The listing builds one solid part. Answer for the finished solid, in the listing's coordinates (mm). A direction names the side the tool comes from. Coordinates: 2 decimals unless noted, no trailing zeros. Order: outer loops, then holes, each group sorted by start corner. A loop starts at its lowest first (then second) coordinate and runs counter-clockwise, first axis right, second up. Notation, with made-up numbers: (68, 47.25) -> (91, 47.25) arc R30 cw to (91, 74.25) -> close; hole circle Ø2 at (7.5, -21). An arc over 180 degrees is marked (long way). Write item = value, one per line. Start each with the question number.
```python
from build123d import *

# Parameters (mm, degrees)
ESQUISSE1_W             = 69
ESQUISSE1_H             = 34
BOSS_EXTRU_1_DEPTH      = 140
COQUE1_T                = 3
CONG_3_R                = 4
ESQUISSE2_W             = 19
ESQUISSE2_H             = 10
ESQUISSE2_R             = 1.75
BOSS_EXTRU_2_DEPTH      = 4
CONG_5_R                = 3.5
ESQUISSE1_2_W           = 69
ESQUISSE1_2_H           = 34
ENL_V_MAT_EXTRU_1_DEPTH = 140
CONG_4_R                = 1
CONG_7_R                = 3
ENL_V_MAT_EXTRU_2_REACH = 155.64
ESQUISSE3_W             = 61
ESQUISSE3_H             = 26
CONG_8_R                = 1


with BuildPart() as part:
    # Esquisse1 → Boss.-Extru.1 (new body)
    with BuildSketch(Plane.XY):
        Rectangle(ESQUISSE1_W, ESQUISSE1_H)
    extrude(amount=BOSS_EXTRU_1_DEPTH)

    # Coque1
    coque1_openings = [part.faces().sort_by_distance(p)[0] for p in [
        (0, 0, 140),
    ]]
    offset(amount=COQUE1_T, openings=coque1_openings, kind=Kind.INTERSECTION)

    # Congé3
    # the kernel refuses this fillet: 4 mm, written as the material it takes off along each edge
    with BuildSketch(Plane(origin=(33.5, 16, 1), x_dir=(0, 1, 0), z_dir=(0, 0, -1))) as cong_3_piece_1_section:
        Polygon((0, 0), (CONG_3_R, 0), (CONG_3_R, CONG_3_R), (0, CONG_3_R), align=None)
    cong_3_piece_1 = extrude(amount=CONG_3_R, mode=Mode.PRIVATE)
    cong_3_piece_1 = cong_3_piece_1 - Plane(origin=(33.5, 16, 1), x_dir=(-0.7071067811865475, -0.7071067811865475, 0), z_dir=(0, 0, -1)) * Sphere(CONG_3_R, mode=Mode.PRIVATE)
    add(cong_3_piece_1, mode=Mode.SUBTRACT)
    with BuildSketch(Plane(origin=(-33.5, 16, 1), x_dir=(0, 0, -1), z_dir=(-1, 0, 0))) as cong_3_piece_2_section:
        Polygon((0, 0), (CONG_3_R, 0), (CONG_3_R, -CONG_3_R), (0, -CONG_3_R), align=None)
    cong_3_piece_2 = extrude(amount=CONG_3_R, mode=Mode.PRIVATE)
    cong_3_piece_2 = cong_3_piece_2 - Plane(origin=(-33.5, 16, 1), x_dir=(0, -0.7071067811865475, 0.7071067811865475), z_dir=(-1, 0, 0)) * Sphere(CONG_3_R, mode=Mode.PRIVATE)
    add(cong_3_piece_2, mode=Mode.SUBTRACT)
    with BuildSketch(Plane(origin=(33.5, -16, 1), x_dir=(0, 0, -1), z_dir=(0, -1, 0))) as cong_3_piece_3_section:
        Polygon((0, 0), (CONG_3_R, 0), (CONG_3_R, CONG_3_R), (0, CONG_3_R), align=None)
    cong_3_piece_3 = extrude(amount=CONG_3_R, mode=Mode.PRIVATE)
    cong_3_piece_3 = cong_3_piece_3 - Plane(origin=(33.5, -16, 1), x_dir=(-0.7071067811865475, 0, 0.7071067811865475), z_dir=(0, -1, 0)) * Sphere(CONG_3_R, mode=Mode.PRIVATE)
    add(cong_3_piece_3, mode=Mode.SUBTRACT)
    with BuildSketch(Plane(origin=(-33.5, -16, 1), x_dir=(-1, 0, 0), z_dir=(0, -1, 0))) as cong_3_piece_4_section:
        Polygon((0, 0), (CONG_3_R, 0), (CONG_3_R, CONG_3_R), (0, CONG_3_R), align=None)
    cong_3_piece_4 = extrude(amount=CONG_3_R, mode=Mode.PRIVATE)
    cong_3_piece_4 = cong_3_piece_4 - Plane(origin=(-33.5, -16, 1), x_dir=(0.7071067811865475, 0, 0.7071067811865475), z_dir=(0, -1, 0)) * Sphere(CONG_3_R, mode=Mode.PRIVATE)
    add(cong_3_piece_4, mode=Mode.SUBTRACT)
    with BuildSketch(Plane(origin=(33.5, 20, -3), x_dir=(0, 0, 1), z_dir=(-1, 0, 0)), Plane(origin=(-33.5, -20, -3), x_dir=(0, 0, 1), z_dir=(1, 0, 0))) as cong_3_piece_5:
        with BuildLine():
            CenterArc((CONG_3_R, -CONG_3_R), CONG_3_R, 90, 90)
            Line((0, -CONG_3_R), (0, 0))
            Line((0, 0), (CONG_3_R, 0))
        make_face()
    extrude(amount=67, mode=Mode.SUBTRACT)
    with BuildSketch(Plane(origin=(37.5, -16, -3), x_dir=(0, 0, 1), z_dir=(0, 1, 0)), Plane(origin=(-37.5, 16, -3), x_dir=(0, 0, 1), z_dir=(0, -1, 0))) as cong_3_piece_6:
        with BuildLine():
            CenterArc((CONG_3_R, -CONG_3_R), CONG_3_R, 90, 90)
            Line((0, -CONG_3_R), (0, 0))
            Line((0, 0), (CONG_3_R, 0))
        make_face()
    extrude(amount=32, mode=Mode.SUBTRACT)
    with BuildSketch(Plane(origin=(-37.5, 20, 1), x_dir=(1, 0, 0), z_dir=(0, 0, 1)), Plane(origin=(37.5, 20, 150), x_dir=(-1, 0, 0), z_dir=(0, 0, -1)), Plane(origin=(37.5, -20, 150), x_dir=(0, 1, 0), z_dir=(0, 0, -1)), Plane(origin=(-37.5, -20, 150), x_dir=(1, 0, 0), z_dir=(0, 0, -1))) as cong_3_piece_7:
        with BuildLine():
            CenterArc((CONG_3_R, -CONG_3_R), CONG_3_R, 90, 90)
            Line((0, -CONG_3_R), (0, 0))
            Line((0, 0), (CONG_3_R, 0))
        make_face()
    extrude(amount=149, mode=Mode.SUBTRACT)

    # Esquisse2 → Boss.-Extru.2 (add)
    # profile 1 of 7: a face of its own
    with BuildSketch(Plane(origin=(0, 20, 0), x_dir=(1, 0, 0), z_dir=(0, 1, 0))):
        with Locations((-43, -33.75)):
            Rectangle(ESQUISSE2_W, ESQUISSE2_H)
        with Locations(Location((-45, -33.75, 0), (0, 0, 270))):
            Circle(ESQUISSE2_R, mode=Mode.SUBTRACT)
    # profile 2 of 7: a face of its own
    with BuildSketch(Plane(origin=(0, 20, 0), x_dir=(1, 0, 0), z_dir=(0, 1, 0))):
        with Locations((-43, -54.625)):
            Rectangle(ESQUISSE2_W, ESQUISSE2_H)
        with Locations(Location((-45, -54.625, 0), (0, 0, 270))):
            Circle(ESQUISSE2_R, mode=Mode.SUBTRACT)
    # profile 3 of 7: a face of its own
    with BuildSketch(Plane(origin=(0, 20, 0), x_dir=(1, 0, 0), z_dir=(0, 1, 0))):
        with Locations((43, -33.75)):
            Rectangle(ESQUISSE2_W, ESQUISSE2_H)
        with Locations(Location((45, -33.75, 0), (0, 0, 270))):
            Circle(ESQUISSE2_R, mode=Mode.SUBTRACT)
    # profile 4 of 7: a face of its own
    with BuildSketch(Plane(origin=(0, 20, 0), x_dir=(1, 0, 0), z_dir=(0, 1, 0))):
        with Locations((-43, -75.5)):
            Rectangle(ESQUISSE2_W, ESQUISSE2_H)
        with Locations(Location((-45, -75.5, 0), (0, 0, 270))):
            Circle(ESQUISSE2_R, mode=Mode.SUBTRACT)
    # profile 5 of 7: a face of its own
    with BuildSketch(Plane(origin=(0, 20, 0), x_dir=(1, 0, 0), z_dir=(0, 1, 0))):
        with Locations((43, -54.625)):
            Rectangle(ESQUISSE2_W, ESQUISSE2_H)
        with Locations(Location((45, -54.625, 0), (0, 0, 270))):
            Circle(ESQUISSE2_R, mode=Mode.SUBTRACT)
    # profile 6 of 7: a face of its own
    with BuildSketch(Plane(origin=(0, 20, 0), x_dir=(1, 0, 0), z_dir=(0, 1, 0))):
        with Locations((-43, -96.375)):
            Rectangle(ESQUISSE2_W, ESQUISSE2_H)
        with Locations(Location((-45, -96.375, 0), (0, 0, 270))):
            Circle(ESQUISSE2_R, mode=Mode.SUBTRACT)
    # profile 7 of 7: a face of its own
    with BuildSketch(Plane(origin=(0, 20, 0), x_dir=(1, 0, 0), z_dir=(0, 1, 0))):
        with Locations((43, -96.375)):
            Rectangle(ESQUISSE2_W, ESQUISSE2_H)
        with Locations(Location((45, -96.375, 0), (0, 0, 270))):
            Circle(ESQUISSE2_R, mode=Mode.SUBTRACT)
    extrude(amount=-BOSS_EXTRU_2_DEPTH)

    # Congé5
    cong_5_edges = [part.edges().sort_by_distance(p)[0] for p in [
        (52.5, 18, 28.75),
        (52.5, 18, 38.75),
        (52.5, 18, 49.625),
        (52.5, 18, 59.625),
        (-52.5, 18, 91.375),
        (-52.5, 18, 101.375),
        (-52.5, 18, 80.5),
        (-52.5, 18, 70.5),
        (52.5, 18, 91.375),
        (52.5, 18, 101.375),
        (-52.5, 18, 28.75),
        (-52.5, 18, 38.75),
        (-52.5, 18, 49.625),
        (-52.5, 18, 59.625),
    ]]
    fillet(cong_5_edges, radius=CONG_5_R)

    # Esquisse1<2> → Enlèv. mat.-Extru.1 (cut)
    with BuildSketch(Plane.XY):
        Rectangle(ESQUISSE1_2_W, ESQUISSE1_2_H)
    extrude(amount=ENL_V_MAT_EXTRU_1_DEPTH, mode=Mode.SUBTRACT)

    # Congé4
    cong_4_edges = [part.edges().sort_by_distance(p)[0] for p in [
        (-34.5, 0, 0),
        (-34.5, 17, 70),
        (0, -17, 0),
        (-34.5, -17, 70),
        (34.5, 0, 0),
        (34.5, -17, 70),
        (0, 17, 0),
        (34.5, 17, 70),
    ]]
    fillet(cong_4_edges, radius=CONG_4_R)

    # Congé7
    # the kernel refuses this fillet: 3 mm, written as the material it adds along each edge
    with BuildSketch(Plane(origin=(37.5, 16, 38.75), x_dir=(0, -1, 0), z_dir=(0, 0, -1)), Plane(origin=(37.5, 16, 59.625), x_dir=(0, -1, 0), z_dir=(0, 0, -1)), Plane(origin=(-37.5, 16, 91.375), x_dir=(0, -1, 0), z_dir=(0, 0, 1)), Plane(origin=(-37.5, 16, 70.5), x_dir=(0, -1, 0), z_dir=(0, 0, 1)), Plane(origin=(37.5, 16, 101.375), x_dir=(0, -1, 0), z_dir=(0, 0, -1)), Plane(origin=(-37.5, 16, 28.75), x_dir=(0, -1, 0), z_dir=(0, 0, 1)), Plane(origin=(-37.5, 16, 49.625), x_dir=(0, -1, 0), z_dir=(0, 0, 1))) as cong_7_piece_1:
        with BuildLine():
            CenterArc((CONG_7_R, -CONG_7_R), CONG_7_R, 90, 90)
            Line((0, -CONG_7_R), (0, 0))
            Line((0, 0), (CONG_7_R, 0))
        make_face()
    extrude(amount=10)

    # Esquisse3 → Enlèv. mat.-Extru.2 (cut, up to next)
    with BuildSketch(Plane(origin=(0, 0, -3), x_dir=(-1, 0, 0), z_dir=(0, 0, -1)), mode=Mode.PRIVATE) as enl_v_mat_extru_2_sk1:
        Rectangle(ESQUISSE3_W, ESQUISSE3_H)
    enl_v_mat_extru_2_tool1 = extrude(enl_v_mat_extru_2_sk1.sketch, amount=-ENL_V_MAT_EXTRU_2_REACH, mode=Mode.PRIVATE) & part.part
    add(enl_v_mat_extru_2_tool1.solids().sort_by_distance((0, 0, -3))[0], mode=Mode.SUBTRACT)

    # Congé8
    cong_8_edges = [part.edges().sort_by_distance(p)[0] for p in [
        (30.5, -13, -1.5),
        (30.5, 13, -1.5),
        (-30.5, 13, -1.5),
        (-30.5, -13, -1.5),
    ]]
    fillet(cong_8_edges, radius=CONG_8_R)


solid = part.part
```
Item 1: For a pull along Z with two mould halves and no side action, classify faces 5 (the flat face through (-43, 18, 28.75)), 6 (the flat face through (52.5, 18, 96)), 7 (the flat face through (-43, 18, 91.375)) as pulls with the +Z half, pulls with the -Z half, needs draft (parallel to the pull), parting line crosses it, or undercut.
Item 2: Which of the six approach directions +Z, -Z, +X, -X, +Y, -Y give full straight-line access (tool end or side, diameter ignored) to faces 1 (the flat face through (46, 16, 53)), 2 (the cylindrical face through (51.448, 17.972, 50.623)), 3 (the flat face through (-30.5, 0, -2)), 4 (the cylindrical face through (-51.502, 17.972, 58.573))?
Item 3: Section B-B, the plane z = 75.5 is taken. Give the vertices of the cut face in (x, y).
Item 4: Section A-A, the plane x = -45 is taken. Give the number of separate pieces and of enclosed holes in the cut face, then the cut area to 3 significant figures.
Item 5: Consider probe 1 along X at (y, z) = (17.7, 33.75); probe 2 along X at (y, z) = (-11, 69); probe 3 along Y at (x, z) = (-1, 34.5). Determine where each line is inside the solid, lowest interval first.
Item 6: Each of these flat-tipped pins is pushed along its axis until it touches: pin 1 (10 mm diameter, centred on x = 9.5, y = -11, fed in from +Z); pin 2 (2 mm diameter, centred on y = -3, z = 23.5, fed in from +X); pin 3 (8 mm diameter, centred on y = -1, z = 95.5, fed in from -X). Where does it stop, or does it pass through?
Item 7: Section C-C, the plane y = -3.5 is taken. Give the vertices of the cut face in (x, z), then the cut area to 3 significant figures.
Item 8: Section D-D, the plane x = -7 is taken. Give the vertices of the cut face in (y, z), then the cut area to 3 significant figures.
A:
q1.face_5 = pulls with the -Z half
q1.face_6 = needs draft
q1.face_7 = undercut
q2.face_1 = +Z, -Z, +X, -Y
q2.face_2 = +X, +Y, -Y
q2.face_3 = +Z, -Z
q2.face_4 = -X, +Y, -Y
q3.outline = (-52.5, 16) -> (-46.75, 16) -> (-46.75, 20) -> (-52.5, 20) -> close; (-43.25, 16) -> (-40.5, 16) arc R3 cw to (-37.5, 13) -> (-37.5, -16) arc R4 ccw to (-33.5, -20) -> (33.5, -20) arc R4 ccw to (37.5, -16) -> (37.5, 16) arc R4 ccw to (33.5, 20) -> (-43.25, 20) -> close; hole (-34.5, -16) arc R1 ccw to (-33.5, -17) -> (33.5, -17) arc R1 ccw to (34.5, -16) -> (34.5, 16) arc R1 ccw to (33.5, 17) -> (-33.5, 17) arc R1 ccw to (-34.5, 16) -> close
q4.separate_pieces = 8
q4.enclosed_holes = 0
q4.area = 104 mm^2
q5.probe_1 = -52.5 to -46.75, -43.25 to 43.25, 46.75 to 52.5
q5.probe_2 = -37.5 to -34.5, 34.5 to 37.5
q5.probe_3 = -20 to -17, 17 to 20
q6.pin_1 = 0
q6.pin_2 = 37.5
q6.pin_3 = -37.5
q7.outline = (-37.5, 1) arc R4 ccw to (-33.5, -3) -> (-30.5, -3) -> (-30.5, 0) -> (-33.5, 0) arc R1 cw to (-34.5, 1) -> (-34.5, 140) -> (-37.5, 140) -> close; (30.5, -3) -> (33.5, -3) arc R4 ccw to (37.5, 1) -> (37.5, 140) -> (34.5, 140) -> (34.5, 1) arc R1 cw to (33.5, 0) -> (30.5, 0) -> close
q7.area = 876 mm^2
q8.outline = (-20, 1) arc R4 ccw to (-16, -3) -> (-13, -3) -> (-13, 0) -> (-16, 0) arc R1 cw to (-17, 1) -> (-17, 140) -> (-20, 140) -> close; (13, -3) -> (16, -3) arc R4 ccw to (20, 1) -> (20, 140) -> (17, 140) -> (17, 1) arc R1 cw to (16, 0) -> (13, 0) -> close
q8.area = 876 mm^2
